Can you work these out from the model? Positions are in its coordinate system, mm. Round coordinates to 2 decimals unless told otherwise and drop trailing zeros. Order: outer loops, then holes, each group sorted by start corner. A loop starts at its lowest first (then second) coordinate and runs counter-clockwise, first axis right, second up. Notation, with made-up numbers: M 76,21 L 110,21 A12 ccw 110,36 Z; hole C -12.5,61 d5. An arc over 180 degrees is marked long. One line per question, with ' | ' between items.
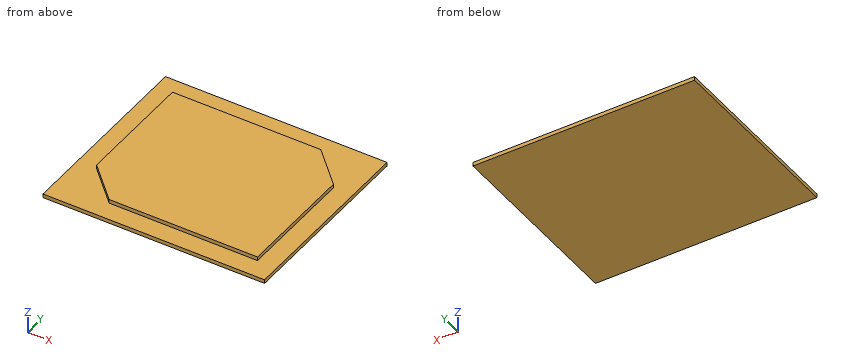
```python
from build123d import *

# Parameters (mm, degrees)
F0_W     = 47.5
F0_H     = 40
F1_DEPTH = 2
F0_W_2   = 57.5
F0_H_2   = 50
F2_DEPTH = 1
F3_SIZE  = 9


with BuildPart() as f1:
    # F0 (on Top) → F1 (new body)
    with BuildSketch(Plane.XY):
        Rectangle(F0_W, F0_H)
    extrude(amount=F1_DEPTH)

    # F0 (on Top) → F2 (join)
    with BuildSketch(Plane.XY):
        Rectangle(F0_W_2, F0_H_2)
        Rectangle(F0_W, F0_H, mode=Mode.SUBTRACT)
    extrude(amount=F2_DEPTH)

    # F3
    f3_edges = [f1.edges().sort_by_distance(p)[0] for p in [
        (-23.75, -20, 1.5),
        (23.75, 20, 1.5),
    ]]
    chamfer(f3_edges, length=F3_SIZE)


solid = f1.part
```
(1) If we section it at A-A on x = 23: Please give me the cut outline in (y, z).
Final values:
outline: M -25,0 L 25,0 L 25,1 L 11.75,1 L 11.75,2 L -20,2 L -20,1 L -25,1 Z
(2) If we section it at B-B on y = 16.5: Please give me the cut outline in (x, z), plus the area to 3 significant figures.
Final values:
outline: M -28.75,0 L 28.75,0 L 28.75,1 L 18.25,1 L 18.25,2 L -23.75,2 L -23.75,1 L -28.75,1 Z | area: 99.5 mm^2
(3) If we section it at C-C on z = 1.3: Please give me the cut outline in (x, y).
Final values:
outline: M -23.75,-11 L -14.75,-20 L 23.75,-20 L 23.75,11 L 14.75,20 L -23.75,20 Z
(4) Will these pins go through, and if not, where does the flat tip stop? pin 1 Ø0.8 at (x, z) = (-12.5, 1.5) entering from +Y; pin 2 Ø0.8 at (y, z) = (-1.5, 1.5) entering from -X.
Final values:
pin 1: y = 20 | pin 2: x = -23.75
(5) Please list where these lines run through material, in increasing order: probe 1 along Y at (x, z) = (11, 1.7); probe 2 along X at (y, z) = (3, 1.75); probe 3 along Z at (x, y) = (24.5, 6.5). Write a range as [from, to].
Final values:
probe 1: [-20, 20] | probe 2: [-23.75, 23.75] | probe 3: [0, 1]
